Input: part model. Units: mm. Frame: model coordinates. Face numbers are marked on the shaded views. A direction names the side the tool comes from. Coordinates: 2 decimals unless noted, no trailing zeros. Write each loop counter-clockwise with the first axis right and the second up, starting at its lowest first coordinate (ties: lowest second). Pieces come first, ordered by that corner, then holes.
from build123d import *

# Parameters (mm, degrees)
F0_W     = 18.415
F0_H     = 13.843
F1_DEPTH = 1.5875
F0_W_2   = 20.6502
F0_H_2   = 49.7587174177
F0_W_3   = 177.8
F0_H_3   = 3.175
F2_DEPTH = 12.7


with BuildPart() as f1:
    # F0 (on Top) → F1 (new body)
    with BuildSketch(Plane.XY):
        with Locations((9.8425, 1.0799015641)):
            Rectangle(F0_W, F0_H)
    extrude(amount=F1_DEPTH)



with BuildPart() as f1b:
    # F0 (on Top) → F1, piece 2 (new body)
    with BuildSketch(Plane.XY):
        Polygon((120.65, -54.8127984359), (120.65, 56.9726015641), (101.6, 56.9726015641), (101.6, 36.3224015641), (4.7498, 36.3224015641), (4.7498, 56.9726015641), (1.5748, 56.9726015641), (1.5748, 33.1474015641), (1.5748, 31.6234015641), (19.05, 31.6234015641), (22.225, 31.2424015641), (101.6, 31.2424015641), (101.6, -29.0825984359), (22.225, -29.0825984359), (19.05, -29.4635984359), (1.6357024433, -29.4635984359), (1.5875, -34.1625984359), (1.5875, -54.8127984359), (4.7625, -54.8127984359), (4.7625, -34.1625984359), (101.6, -34.1625984359), (101.6, -54.8127984359), align=None)
        Polygon((-38.1, 56.9726015641), (-57.15, 56.9726015641), (-57.15, -54.8127984359), (-38.1, -54.8127984359), (-38.1, -34.1625984359), (-18.415, -34.1625984359), (-18.415, 36.3224015641), (-38.1, 36.3224015641), align=None)
        with Locations((-31.9151, -1.256839727)):
            Rectangle(F0_W_2, F0_H_2, mode=Mode.SUBTRACT)
        Polygon((-38.1, -54.8127984359), (-57.15, -54.8127984359), (-57.15, -57.9877984359), (120.65, -57.9877984359), (120.65, -54.8127984359), (101.6, -54.8127984359), (4.7625, -54.8127984359), (1.5875, -54.8127984359), align=None)
        Polygon((120.65, 60.1476015641), (-57.15, 60.1476015641), (-57.15, 56.9726015641), (-38.1, 56.9726015641), (1.5748, 56.9726015641), (4.7498, 56.9726015641), (101.6, 56.9726015641), (120.65, 56.9726015641), align=None)
    extrude(amount=F1_DEPTH)


with BuildPart() as f1_1:
    add(f1.part)

    add(f1b.part)  # F2 merges F1b
    # F0 (on Top) → F2 (join)
    with BuildSketch(Plane.XY):
        Polygon((22.225, 31.2424015641), (19.05, 31.6234015641), (19.05, 8.0014015641), (19.05, -5.8415984359), (19.05, -29.4635984359), (22.225, -29.0825984359), align=None)
        with Locations((31.75, -59.5752984359)):
            Rectangle(F0_W_3, F0_H_3)
        with Locations((31.75, 61.7351015641)):
            Rectangle(F0_W_3, F0_H_3)
    extrude(amount=F2_DEPTH)


solid = f1_1.part
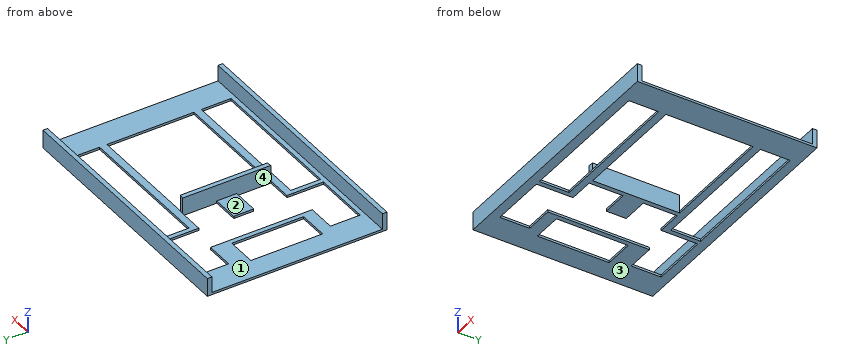
Item 1: Pull-direction query (Y, two-part tool) for the marked faces 3 and 4; classes: released by +Y, released by -Y, zero draft, split by the parting line, or undercut.
Item 2: Material intervals for line 1 (Y direction, x = 53, z = 1); line 2 (Y direction, x = 55.5, z = 9); line 3 (Z direction, x = 51, y = -31.5), sorted ascending.
Item 3: Section query C-C, the plane x = 33. Return loops of the section in (y, z), then the cut area to 3 significant figures.
Item 4: Section query D-D, the plane y = 5. State how many separate pieces and enclosed holes the cut face has, then the cut area to 3 significant figures.
Item 5: Section query A-A, the plane y = -42.5. Return loops of the section in (x, z).
Item 6: Access query for the marked faces 1 and 2. Directions: +Z, -Z, +X, -X, +Y, -Y. A direction counts if a zero-diameter tool reaches every point of the face in a straight line with its end or side. Return the directions, or none.
Item 7: Pin query (flat end, axial travel): pin 1 Ø1 at (x, y) = (101.5, 42.5) entering from +Z; pin 2 Ø3 at (y, z) = (23.5, 7) entering from +X (3 decimals); pin 3 Ø6 at (y, z) = (-33, 10) entering from -X. Return the tip coordinate at first contact, or that it passes through.
Item 8: Section query B-B, the plane z = 6.5. Return loops of the section in (x, y) (3 decimals), then the cut area to 3 significant figures.
The answers:
1. face 3: zero draft
1. face 4: undercut
2. line 1: y = -61.16 to -54.81, -34.16 to -29.08, 31.24 to 36.32, 56.97 to 63.32
2. line 2: y = -61.16 to -57.99, 60.15 to 63.32
2. line 3: z = 0 to 1.59
3. outline: (-61.16, 0) - (-54.81, 0) - (-54.81, 1.59) - (-57.99, 1.59) - (-57.99, 12.7) - (-61.16, 12.7) - close; (-34.16, 0) - (-29.08, 0) - (-29.08, 1.59) - (-34.16, 1.59) - close; (31.24, 0) - (36.32, 0) - (36.32, 1.59) - (31.24, 1.59) - close; (56.97, 0) - (63.32, 0) - (63.32, 12.7) - (60.15, 12.7) - (60.15, 1.59) - (56.97, 1.59) - close
3. area: 107 mm2
4. separate pieces: 4
4. enclosed holes: 0
4. area: 129 mm2
5. outline: (-57.15, 0) - (-38.1, 0) - (-38.1, 1.59) - (-57.15, 1.59) - close; (1.59, 0) - (4.76, 0) - (4.76, 1.59) - (1.59, 1.59) - close; (101.6, 0) - (120.65, 0) - (120.65, 1.59) - (101.6, 1.59) - close
6. face 1: +Z
6. face 2: +Z, -X
7. pin 1: stops at z = 1.59
7. pin 2: stops at x = 22.225
7. pin 3: passes through
8. outline: (-57.15, -61.163) - (120.65, -61.163) - (120.65, -57.988) - (-57.15, -57.988) - close; (-57.15, 60.148) - (120.65, 60.148) - (120.65, 63.323) - (-57.15, 63.323) - close; (19.05, -29.464) - (22.225, -29.083) - (22.225, 31.242) - (19.05, 31.623) - close
8. area: 1,320 mm2
